from build123d import *

# Parameters (mm, degrees)
F1_DEPTH = 10
F3_DEPTH = 5
F4_W     = 15
F4_H     = 30
F5_DEPTH = 5
F6_D     = 6.6
F6_DEPTH = 14.25
F6_TIP   = 1.9828400428


# Not quite as in the source:
# - a pattern or mirror of a feature is missing from the dataset's text; its kind, count and spacing are read off the source's solid


with BuildPart() as f1:
    # F0 (on Front) → F1 (new body)
    with BuildSketch(Plane.XZ):
        with BuildLine():
            ThreePointArc((40, 40), (0, 0), (-40, 40))
            Line((-40, 40), (-85, 40))
            Line((-85, 40), (-85, -60))
            Line((-85, -60), (85, -60))
            Line((85, -60), (85, 40))
            Line((85, 40), (40, 40))
        make_face()
    extrude(amount=F1_DEPTH)

    # F2 (on face) → F3 (join)
    with BuildSketch(Plane(origin=(0, 0, 0), x_dir=(-1, 0, 0), z_dir=(0, 1, 0))):
        with BuildLine():
            ThreePointArc((40, 40), (0, 0), (-40, 40))
            Line((-40, 40), (-85, 40))
            Line((-85, 40), (-85, -60))
            Line((-85, -60), (85, -60))
            Line((85, -60), (85, 40))
            Line((85, 40), (40, 40))
        make_face()
        with BuildLine():
            ThreePointArc((35, 40), (0, 5), (-35, 40))
            Line((-35, 40), (-40, 40))
            ThreePointArc((-40, 40), (0, 0), (40, 40))
            Line((40, 40), (35, 40))
        make_face()
    extrude(amount=F3_DEPTH)

    # F4 (on face) → F5 (join)
    with BuildSketch(Plane.YZ.offset(85)):
        with Locations((-17.5, -45)):
            Rectangle(F4_W, F4_H)
        with Locations((-17.5, -10)):
            Rectangle(F4_W, F4_H)
        with Locations((-17.5, 25)):
            Rectangle(F4_W, F4_H)
    f5 = extrude(amount=-F5_DEPTH)

    # F5_copies: F5 across plane
    add(f5.mirror(Plane(origin=(0, 0, 0), x_dir=(0, 0, -1), z_dir=(-1, 0, 0))))

    # F6
    with Locations(Plane.YZ.offset(85)):
        with Locations((-17.5, 25), (-17.5, -10), (-17.5, -45)):
            f6 = Hole(F6_D / 2, depth=F6_DEPTH)
            with Locations((0, 0, -(F6_DEPTH + F6_TIP / 2))):  # 118° drill point
                Cone(0, F6_D / 2, F6_TIP, mode=Mode.SUBTRACT)

    # F6_copies: F6 across plane
    add(f6.mirror(Plane(origin=(0, 0, 0), x_dir=(0, 0, -1), z_dir=(-1, 0, 0))), mode=Mode.SUBTRACT)


solid = f1.part
Input: part model. Units: mm. Frame: model coordinates. A direction names the side the tool comes from. Round coordinates to 2 decimals unless told otherwise and drop trailing zeros. Order: outer loops, then holes, each group sorted by start corner. A loop starts at its lowest first (then second) coordinate and runs counter-clockwise, first axis right, second up. Notation, with made-up numbers: (68.25, 25) - (78.25, 25) arc R16 ccw to (78.25, 52) - close; hole circle Ø6 at (28.25, 88.25). An arc over 180 degrees is marked (long way). Use a Markdown table: item, result.
1. Access query for faces 1 (the face through (-6, 0, 5)), 2 (the face through (-83, -18, 10)), 3 (the face through (80, -18, -41)), 4 (the face through (83, -25, 25)). Directions: +Z, -Z, +X, -X, +Y, -Y. A direction counts if a zero-diameter tool reaches every point of the face in a straight line with its end or side. Return the directions, or none.
Evaluation:
| item | result |
|---|---|
| face 1 | +Z, -Y |
| face 2 | +X, -X, -Y |
| face 3 | +Z, -Z, -Y |
| face 4 | +Z, -Z, +X, -X, -Y |
2. Mould query, pull axis Z, two halves, no side actions, for faces 5 (the face through (83, -18, -30)), 6 (the face through (0.88, -4.93, 0.01)), 7 (the face through (-80, -21, -10)). Classes: +Z half, -Z half, draft (parallel to the pull), parting line (faces both ways), or undercut.
Evaluation:
| item | result |
|---|---|
| face 5 | undercut |
| face 6 | +Z half |
| face 7 | draft |
3. Section B-B on z = 25. Return the cut outline in (x, y), then the cut area to 3 significant figures.
Evaluation:
| item | result |
|---|---|
| outline | (-85, -25) - (-80, -25) - (-80, -20.8) - (-85, -20.8) - close; (-85, -14.2) - (-80, -14.2) - (-80, -10) - (-37.08, -10) - (-37.08, 0) - (-31.62, 0) - (-31.62, 5) - (-85, 5) - close; (31.62, 0) - (37.08, 0) - (37.08, -10) - (80, -10) - (80, -14.2) - (85, -14.2) - (85, 5) - (31.62, 5) - close; (80, -25) - (85, -25) - (85, -20.8) - (80, -20.8) - close |
| area | 1,580 mm^2 |
4. Section D-D on z = -20. Return the cut outline in (x, y).
Evaluation:
| item | result |
|---|---|
| outline | (-85, -25) - (-80, -25) - (-80, -10) - (80, -10) - (80, -25) - (85, -25) - (85, 5) - (-85, 5) - close |
5. First-contact query: pin 1 (6 mm diameter, centred on y = -17.5, z = 25, fed in from -X); pin 2 (5 mm diameter, centred on x = 41.5, z = -35, fed in from -Y). Flat tips, straight axial feed; report the tip coordinate or a pass-through.
Evaluation:
| item | result |
|---|---|
| pin 1 | through |
| pin 2 | y = -10 |
6. Section A-A on z = -10. Return the cut outline in (x, y), then the cut area to 3 significant figures.
Evaluation:
| item | result |
|---|---|
| outline | (-85, -25) - (-80, -25) - (-80, -20.8) - (-85, -20.8) - close; (-85, -14.2) - (-80, -14.2) - (-80, -10) - (80, -10) - (80, -14.2) - (85, -14.2) - (85, 5) - (-85, 5) - close; (80, -25) - (85, -25) - (85, -20.8) - (80, -20.8) - close |
| area | 2,630 mm^2 |
7. Section C-C on x = 0. Return the cut outline in (y, z), then the cut area to 3 significant figures.
Evaluation:
| item | result |
|---|---|
| outline | (-10, -60) - (5, -60) - (5, 5) - (0, 5) - (0, 0) - (-10, 0) - close |
| area | 925 mm^2 |
8. Material intervals for probe 1 along Z at (x, y) = (81.95, -17.5); probe 2 along Y at (x, z) = (-83.5, -10); probe 3 along X at (y, z) = (-22.25, 35), sorted ascending.
Evaluation:
| item | result |
|---|---|
| probe 1 | -60 to -48.3, -41.7 to -30, -25 to -13.3, -6.7 to 5, 10 to 21.7, 28.3 to 40 |
| probe 2 | -25 to -20.8, -14.2 to 5 |
| probe 3 | -85 to -80, 80 to 85 |
